Read the model definition and answer for the solid it produces. Units are mm, in the model's axes. A direction names the side the tool comes from. Coordinates: 2 decimals unless noted, no trailing zeros. Order: outer loops, then holes, each group sorted by start corner. A loop starts at its lowest first (then second) coordinate and runs counter-clockwise, first axis right, second up.
```python
from build123d import *

# Parameters (mm, degrees)
F1_DEPTH = 5
F3_DEPTH = 15
F4_D     = 5.5
F4_DEPTH = 13.5
F4_TIP   = 1.6523667023


with BuildPart() as f1:
    # F0 (on Top) → F1 (new body)
    with BuildSketch(Plane.XY):
        Polygon((42.5, 30), (-42.5, 30), (-42.5, 0), (-18.5, -30), (18.5, -30), (42.5, 0), align=None)
    extrude(amount=F1_DEPTH)

    # F2 (on Top) → F3 (join)
    with BuildSketch(Plane.XY):
        with BuildLine():
            ThreePointArc((21.5, 0), (0, -21.5), (-21.5, 0))
            Line((-21.5, 0), (-28.5, 0))
            ThreePointArc((-28.5, 0), (0, -28.5), (28.5, 0))
            Line((28.5, 0), (21.5, 0))
        make_face()
    extrude(amount=F3_DEPTH)

    # F4
    with Locations(Plane(origin=(0, 0, 0), x_dir=(1, 0, 0), z_dir=(0, 0, -1))):
        with Locations((-34.5, -22), (34.5, -22)):
            Hole(F4_D / 2, depth=F4_DEPTH)
            with Locations((0, 0, -(F4_DEPTH + F4_TIP / 2))):  # 118° drill point
                Cone(0, F4_D / 2, F4_TIP, mode=Mode.SUBTRACT)


solid = f1.part
```
1) Which of the six approach directions +Z, -Z, +X, -X, +Y, -Y give full straight-line access (tool end or side, diameter ignored) to faces 4 (the flat face through (0, -30, 2)), 5 (the cylindrical face through (-0.627, -28.493, 9.93)), 6 (the flat face through (25, 0, 10))?
A:
face 4: +Z, -Z, +X, -X, -Y
face 5: +Z, -Y
face 6: +Z, +X, -X, +Y
2) A cutting plane is placed at C-C, the plane x = 0. Determine the outline of the cut face in (y, z).
A:
outline: (-30, 0) - (30, 0) - (30, 5) - (-21.5, 5) - (-21.5, 15) - (-28.5, 15) - (-28.5, 5) - (-30, 5) - close
3) Straight lines are drawn through the part: line 1 (X direction, y = 22, z = 2.1); line 2 (Z direction, x = -14.5, y = -10); line 3 (Y direction, x = -34.5, z = 3.95). For each, find the intervals that lie inside material, in ascending order.
A:
line 1: x = -42.5 to -37.25, -31.75 to 31.75, 37.25 to 42.5
line 2: z = 0 to 5
line 3: y = -10 to 19.25, 24.75 to 30
4) A cutting plane is placed at B-B, the plane y = 22. Determine the outline of the cut face in (x, z), and give its area (3 significant figures).
A:
outline: (-42.5, 0) - (-37.25, 0) - (-37.25, 5) - (-42.5, 5) - close; (-31.75, 0) - (31.75, 0) - (31.75, 5) - (-31.75, 5) - close; (37.25, 0) - (42.5, 0) - (42.5, 5) - (37.25, 5) - close
area: 370 mm2
5) Determine the mould class of faces 1 (the flat face through (42.5, 15, 2)), 2 (the cylindrical face through (0.473, -21.495, 9.93)), 3 (the cylindrical face through (-31.753, 21.879, 2.535)) for opening direction Y: pulls with the +Y half, pulls with the -Y half, needs draft (parallel to the pull), parting line crosses it, or undercut.
A:
face 1: needs draft
face 2: pulls with the +Y half
face 3: undercut
6) A cutting plane is placed at D-D, the plane z = 12.5. Determine the outline of the cut face in (x, y).
A:
outline: (-28.5, 0) arc R28.5 ccw to (28.5, 0) - (21.5, 0) arc R21.5 cw to (-21.5, 0) - close
7) A cutting plane is placed at A-A, the plane x = 34.5. Determine the outline of the cut face in (y, z).
A:
outline: (-10, 0) - (19.25, 0) - (19.25, 5) - (-10, 5) - close; (24.75, 0) - (30, 0) - (30, 5) - (24.75, 5) - close
8) Flat-ended cylindrical pins translate along their axes: pin 1 Ø3 at (y, z) = (-21.5, 2) entering from -X; pin 2 Ø6 at (x, z) = (2, 10.5) entering from -Y; pin 3 Ø7.5 at (x, z) = (24, 10) entering from +Y. Find the tip coordinate at first contact, or state that the pin passes through.
A:
pin 1: stops at x = -26.5
pin 2: stops at y = -28.5
pin 3: stops at y = 0
